Could you check a few things on this model? Use its own coordinates, in mm. A direction names the side the tool comes from. Give positions to 0.01 mm unless a question says otherwise; leave off trailing zeros. Loops run counter-clockwise (first coordinate to the right, second up) from the corner with the lowest first, then second, coordinate; pieces in that order, holes last. Notation, with made-up numbers: M 30.5,18 L 69.5,18 A25 ccw 69.5,37 Z; hole C -15,-39.5 d2. An arc over 180 degrees is marked long. Return JSON: item names as keys, results as strings. Group by question number.
1. If we section it at A-A (z = -107.5): Write out the boundary of the cut face in (x, y).
2. If we section it at C-C (y = 74.5): Write out the boundary of the cut face in (x, z).
3. If we section it at D-D (x = 10): Write out the boundary of the cut face in (y, z), plus the area to 3 significant figures.
4. For pin 1 (12 mm diameter, centred on y = 146, z = -72, fed in from -X); pin 2 (12 mm diameter, centred on x = -1.5, z = -104.5, fed in from -Y); pin 3 (3 mm diameter, centred on y = 65.5, z = -68.5, fed in from -X), each with a flat end and sliding along its axis, tell me the tip position at first contact or that it passes through.
5. If we section it at B-B (x = -88.5): Write out the boundary of the cut face in (y, z), plus the area to 3 significant figures.
6. Please list where these lines run through material, in increasing order: line 1 (X direction, y = 104, z = -79); line 2 (Y direction, x = -152, z = -80); line 3 (X direction, y = 97.5, z = -73.5).
7. For faces 5 (the flat face through (75, 105, -80)), 6 (the cylindrical face through (126.71, 133.88, -78.18)), 7 (the cylindrical face through (-8.13, 79.22, -43.39)), 8 (the flat face through (-77, 103.858, -79.475)), which set-ups out of +Z, -Z, +X, -X, +Y, -Y let a thin tool reach every point of the face, with its end or its side?
8. If we mould it in two halves opening along X, with no side actions, what happens to faces 1 (the flat face through (77, 103.858, -79.475)), 2 (the cylindrical face through (-37.495, 106.634, -80.632)), 3 (the flat face through (-75, 105, -80)), 4 (the cylindrical face through (-126.71, 133.88, -78.18))? For each: +X half, -X half, draft (parallel to the pull), parting line (faces both ways), or undercut.
```python
from build123d import *

# Parameters (mm, degrees)
SKETCH_1_R          = 37.5
SKETCH_1_R_2        = 35
SKETCH_4_R          = 37.5
SKETCH_4_R_2        = 35
EXTRUDE_1_DEPTH     = 75
EXTRUDE_START       = 2
SKETCH_5_R          = 37.5
SKETCH_5_R_2        = 14
EXTRUDE_2_DEPTH     = 2
EXTRUDE_START_2     = 100
SKETCH_6_R          = 16
SKETCH_6_R_2        = 14
EXTRUDE_3_DEPTH     = 100
SKETCH_7_W          = 164.087293052
SKETCH_7_H          = 105
CUT_EXTRUDE_1_DEPTH = 265.464553435


with BuildPart() as part:
    # 扫描2: sweep along a path in 草图2
    with BuildLine(Plane(origin=(0, 0, 0), x_dir=(0, 0, -1), z_dir=(1, 0, 0))) as sweep_2_path:
        Line((0, 0), (40, 0))
        ThreePointArc((40, 0), (68.284271247, 11.715728753), (80, 40))
        Line((80, 40), (80, 120))
    # 草图1 → 扫描2 (sweep)
    with BuildSketch(Plane.XY):
        Circle(SKETCH_1_R)
        Circle(SKETCH_1_R_2, mode=Mode.SUBTRACT)
    sweep(path=sweep_2_path.line)

    # 草图4 → 凸台-拉伸1 (add, symmetric)
    with BuildSketch(Plane(origin=(0, 0, 0), x_dir=(0, 0, -1), z_dir=(1, 0, 0))):
        with Locations((80, 120)):
            Circle(SKETCH_4_R)
        with Locations((80, 120)):
            Circle(SKETCH_4_R_2, mode=Mode.SUBTRACT)
    extrude(amount=EXTRUDE_1_DEPTH, both=True)

    # 草图5 → 凸台-拉伸2 (add)
    with BuildSketch(Plane(origin=(75, 0, 0), x_dir=(0, 0, -1), z_dir=(1, 0, 0)).offset(EXTRUDE_START)):
        with Locations((80, 120)):
            Circle(SKETCH_5_R)
        with Locations((80, 120)):
            Circle(SKETCH_5_R_2, mode=Mode.SUBTRACT)
    extrude_2 = extrude(amount=-EXTRUDE_2_DEPTH)

    # 草图6 → 凸台-拉伸3 (add)
    with BuildSketch(Plane(origin=(77, 0, 0), x_dir=(0, 0, -1), z_dir=(1, 0, 0)).offset(EXTRUDE_START_2)):
        with Locations((80, 120)):
            Circle(SKETCH_6_R)
        with Locations((80, 120)):
            Circle(SKETCH_6_R_2, mode=Mode.SUBTRACT)
    extrude_3 = extrude(amount=-EXTRUDE_3_DEPTH)

    # 镜向1: 凸台-拉伸2, 凸台-拉伸3 across plane
    add(extrude_2.mirror(Plane(origin=(0, 0, 0), x_dir=(0, 0, 1), z_dir=(1, 0, 0))))
    add(extrude_3.mirror(Plane(origin=(0, 0, 0), x_dir=(0, 0, 1), z_dir=(1, 0, 0))))

    # 草图7 → 切除-拉伸1 (cut, through all)
    with BuildSketch(Plane.XY):
        Rectangle(SKETCH_7_W, SKETCH_7_H)
    extrude(amount=-CUT_EXTRUDE_1_DEPTH, mode=Mode.SUBTRACT)


solid = part.part
```
Answer:
{
 "1": {"outline": "M -77,94.5 L -25.5,94.5 L -25.5,52.5 L -21.65,52.5 L -21.65,94.5 L 21.65,94.5 L 21.65,52.5 L 25.5,52.5 L 25.5,94.5 L 77,94.5 L 77,145.5 L -77,145.5 Z; hole M -75,98.35 L -25.5,98.35 L -25.5,120 L -21.65,120 L -21.65,98.35 L 21.65,98.35 L 21.65,120 L 25.5,120 L 25.5,98.35 L 75,98.35 L 75,141.65 L -75,141.65 Z"},
 "2": {"outline": "C 0,-80 d75; hole C 0,-80 d70"},
 "3": {"outline": "M 52.5,-116.14 L 110,-116.14 A37.5 ccw long 110,-43.86 L 52.5,-43.86 L 52.5,-46.46 L 103.23,-46.46 A37.5 ccw 103.23,-113.54 L 52.5,-113.54 Z; hole M 110,-113.54 L 120,-113.54 L 120,-115 A35 ccw 120,-45 L 120,-46.46 L 110,-46.46 A35 ccw Z", "area": "869 mm²"},
 "4": {"pin 1": "stops at x = -77", "pin 2": "stops at y = 87.38", "pin 3": "stops at x = -36.14"},
 "5": {"outline": "C 120,-80 d32; hole C 120,-80 d28", "area": "188 mm²"},
 "6": {"line 1": "x = -77 to -75, -37.49 to -34.99, 34.99 to 37.49, 75 to 77", "line 2": "y = 104 to 106, 134 to 136", "line 3": "x = -77 to -75, -36.93 to -34.39, 34.39 to 36.93, 75 to 77"},
 "7": {"face 5": "none", "face 6": "+X", "face 7": "-Y", "face 8": "-X"},
 "8": {"face 1": "+X half", "face 2": "undercut", "face 3": "undercut", "face 4": "draft"}
}
